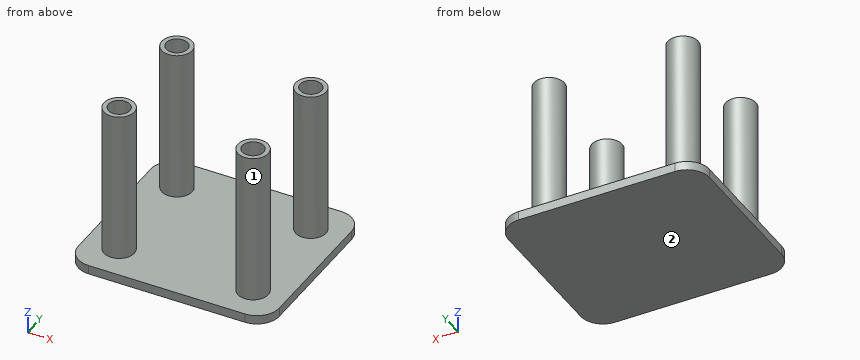
```python
from build123d import *

# Parameters (mm, degrees)
F0_W     = 45
F0_H     = 40
F1_DEPTH = 2
F2_R     = 3.4
F3_DEPTH = 34
F4_R     = 2.4
F5_DEPTH = 30
F6_R     = 5


with BuildPart() as f1:
    # F0 (on Top) → F1 (new body)
    with BuildSketch(Plane.XY):
        Rectangle(F0_W, F0_H)
    extrude(amount=F1_DEPTH)

    # F2 (on face) → F3 (join)
    with BuildSketch(Plane.XY.offset(2)):
        with Locations((-15, 12)):
            Circle(F2_R)
        with Locations((15, 12)):
            Circle(F2_R)
        with Locations((15, -12)):
            Circle(F2_R)
        with Locations((-15, -12)):
            Circle(F2_R)
    extrude(amount=F3_DEPTH)

    # F4 (on face) → F5 (cut)
    with BuildSketch(Plane.XY.offset(36)):
        with Locations((-15, 12)):
            Circle(F4_R)
        with Locations((15, 12)):
            Circle(F4_R)
        with Locations((15, -12)):
            Circle(F4_R)
        with Locations((-15, -12)):
            Circle(F4_R)
    extrude(amount=-F5_DEPTH, mode=Mode.SUBTRACT)

    # F6
    f6_edges = [f1.edges().sort_by_distance(p)[0] for p in [
        (-22.5, -20, 1),
        (22.5, -20, 1),
        (22.5, 20, 1),
        (-22.5, 20, 1),
    ]]
    fillet(f6_edges, radius=F6_R)


solid = f1.part
```
Model file for the job. Use its own axes, mm. Face numbers are marked on the shaded views. Give positions to 0.01 mm unless a question says otherwise; leave off trailing zeros. Order: outer loops, then holes, each group sorted by start corner. A loop starts at its lowest first (then second) coordinate and runs counter-clockwise, first axis right, second up.
1) Mould opens along X. For the marked faces 1 and 2 say: +X half, -X half, draft (parallel to the pull), parting line (faces both ways), or undercut.
2) Saw through at D-D, the plane y = -0.5. Write the cut outline in (x, z), then the cut area to 3 significant figures.
3) Saw through at A-A, the plane z = 16. Write the cut outline in (x, y).
4) Wall check: probe 1 along Y at (x, z) = (15, 19); probe 2 along X at (y, z) = (11, 29.5); probe 3 along Y at (x, z) = (14, 15). Give the ranges that are in metal, low to high.
5) Saw through at C-C, the plane x = 15. Write the cut outline in (y, z).
6) Pin check, flat tips, straight feed: pin 1 (7.5 mm diameter, centred on x = -15, y = 12, fed in from -Z); pin 2 (1.5 mm diameter, centred on x = -12, z = 16.5, fed in from +Y); pin 3 (1.5 mm diameter, centred on y = 14.5, z = 17, fed in from +X); pin 4 (2.5 mm diameter, centred on x = -15, y = 11.5, fed in from +Z). Stop position of each tip, or through.
7) Saw through at B-B, the plane y = -12. Write the cut outline in (x, z).
Computed:
1. face 1: undercut
1. face 2: draft
2. outline: (-22.5, 0) - (22.5, 0) - (22.5, 2) - (-22.5, 2) - close
2. area: 90.0 mm2
3. outline: circle Ø6.8 at (-15, -12); circle Ø6.8 at (-15, 12); circle Ø6.8 at (15, -12); circle Ø6.8 at (15, 12); hole circle Ø4.8 at (-15, -12); hole circle Ø4.8 at (-15, 12); hole circle Ø4.8 at (15, -12); hole circle Ø4.8 at (15, 12)
4. probe 1: y = -15.4 to -14.4, -9.6 to -8.6, 8.6 to 9.6, 14.4 to 15.4
4. probe 2: x = -18.25 to -17.18, -12.82 to -11.75, 11.75 to 12.82, 17.18 to 18.25
4. probe 3: y = -15.25 to -14.18, -9.82 to -8.75, 8.75 to 9.82, 14.18 to 15.25
5. outline: (-20, 0) - (20, 0) - (20, 2) - (15.4, 2) - (15.4, 36) - (14.4, 36) - (14.4, 6) - (9.6, 6) - (9.6, 36) - (8.6, 36) - (8.6, 2) - (-8.6, 2) - (-8.6, 36) - (-9.6, 36) - (-9.6, 6) - (-14.4, 6) - (-14.4, 36) - (-15.4, 36) - (-15.4, 2) - (-20, 2) - close
6. pin 1: stops at z = 0
6. pin 2: stops at y = 14.55
6. pin 3: stops at x = 17.92
6. pin 4: stops at z = 6
7. outline: (-22.5, 0) - (22.5, 0) - (22.5, 2) - (18.4, 2) - (18.4, 36) - (17.4, 36) - (17.4, 6) - (12.6, 6) - (12.6, 36) - (11.6, 36) - (11.6, 2) - (-11.6, 2) - (-11.6, 36) - (-12.6, 36) - (-12.6, 6) - (-17.4, 6) - (-17.4, 36) - (-18.4, 36) - (-18.4, 2) - (-22.5, 2) - close
